Drawing for the job (mm, zero at the part's lowest x, y, z). Coordinates: 2 decimals unless noted, no trailing zeros. Order: outer loops, then holes, each group sorted by start corner. A loop starts at its lowest first (then second) coordinate and runs counter-clockwise, first axis right, second up. Notation, with made-up numbers: (83, 4) -> (93, 4) arc R30 ccw to (93, 31) -> close; hole circle Ø9 at (38, 25.5). An arc over 180 degrees is marked (long way). Write each question's results on one line, items separated by ' | '.
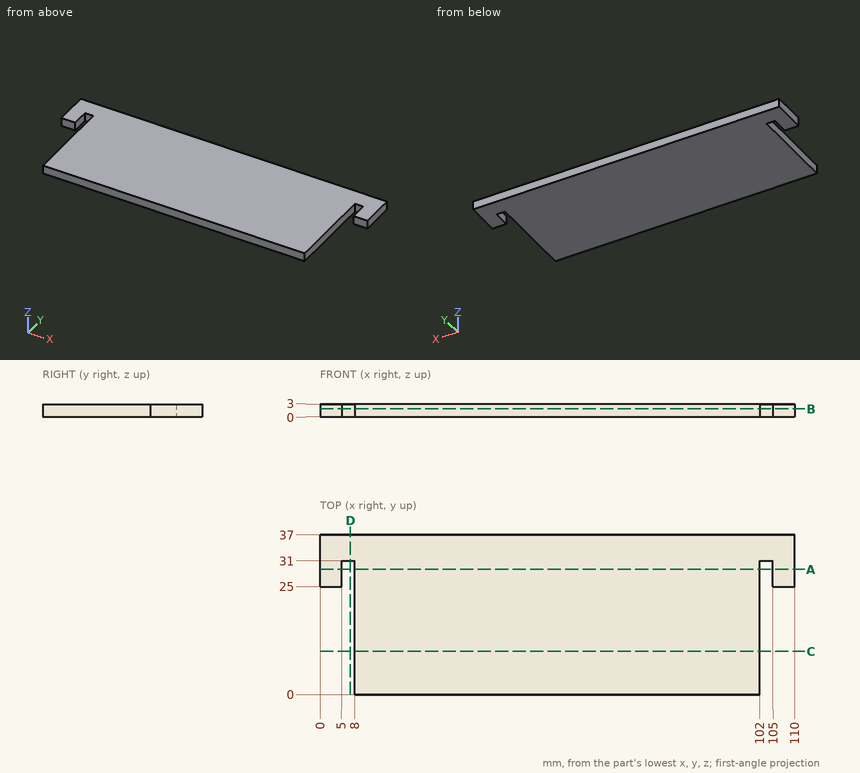
Item 1: Slice it at D-D, the plane x = 7. List the corners of the cut face in (y, z).
Answer:
outline: (31, 0) -> (37, 0) -> (37, 3) -> (31, 3) -> close
Item 2: Drill centre lines: line 1 (X direction, y = 30, z = 2.85); line 2 (Y direction, x = 103, z = 2.1); line 3 (X direction, y = 13, z = 1.95). Where is each one in solid material? Low to high. Write a range as from..to.
Answer:
line 1: x = 0..5, 8..102, 105..110 | line 2: y = 31..37 | line 3: x = 8..102
Item 3: Slice it at C-C, the plane y = 10. List the corners of the cut face in (x, z).
Answer:
outline: (8, 0) -> (102, 0) -> (102, 3) -> (8, 3) -> close
Item 4: Slice it at A-A, the plane y = 29. List the corners of the cut face in (x, z).
Answer:
outline: (0, 0) -> (5, 0) -> (5, 3) -> (0, 3) -> close; (8, 0) -> (102, 0) -> (102, 3) -> (8, 3) -> close; (105, 0) -> (110, 0) -> (110, 3) -> (105, 3) -> close
Item 5: Slice it at B-B, the plane z = 1.85. List the corners of the cut face in (x, y).
Answer:
outline: (0, 25) -> (5, 25) -> (5, 31) -> (8, 31) -> (8, 0) -> (102, 0) -> (102, 31) -> (105, 31) -> (105, 25) -> (110, 25) -> (110, 37) -> (0, 37) -> close
Item 6: Pin check, flat tips, straight feed: pin 1 (1.5 mm diameter, centred on x = 2, z = 2, fed in from -Y); pin 2 (0.9 mm diameter, centred on x = 103, z = 2, fed in from -Y). Stop position of each tip, or through.
Answer:
pin 1: stops at y = 25 | pin 2: stops at y = 31
